```python
from build123d import *

# Parameters (mm, degrees)
SKETCH3_W           = 140
SKETCH3_H           = 140
BOSS_EXTRUDE1_DEPTH = 5
CUT_EXTRUDE1_DEPTH  = 5
CIRPATTERN1_COUNT   = 4
CUT_EXTRUDE2_REACH  = 101.121
SKETCH7_R           = 11
CIRPATTERN2_COUNT   = 4
CIRPATTERN3_COUNT   = 4


with BuildPart() as part:
    # Sketch3 → Boss-Extrude1 (new body)
    with BuildSketch(Plane.XY):
        Rectangle(SKETCH3_W, SKETCH3_H)
    extrude(amount=BOSS_EXTRUDE1_DEPTH)

    # Sketch4 → Cut-Extrude1 (cut)
    with BuildSketch(Plane.XY.offset(5)):
        with BuildLine():
            Line((7.583144073, 14.654211885), (52.928932188, 60))
            Line((52.928932188, 60), (-54.688394727, 60))
            Line((-54.688394727, 60), (-7.80758307, 14.53587447))
            ThreePointArc((-7.80758307, 14.53587447), (-0.126862728, 16.499512291), (7.583144073, 14.654211885))
        make_face()
    cut_extrude1 = extrude(amount=-CUT_EXTRUDE1_DEPTH, mode=Mode.SUBTRACT)

    # CirPattern1: Cut-Extrude1 ×4 about axis
    cirpattern1_axis = Axis((0, 0, 0), (0, 0, 1))
    for i in range(1, CIRPATTERN1_COUNT):
        add(cut_extrude1.rotate(cirpattern1_axis, i * 360 / CIRPATTERN1_COUNT), mode=Mode.SUBTRACT)

    # Sketch7 → Cut-Extrude2 (cut, up to next)
    with BuildSketch(Plane.XY.offset(5), mode=Mode.PRIVATE) as cut_extrude2_sk1:
        Circle(SKETCH7_R)
    cut_extrude2_tool1 = extrude(cut_extrude2_sk1.sketch, amount=-CUT_EXTRUDE2_REACH, mode=Mode.PRIVATE) & part.part
    add(cut_extrude2_tool1.solids().sort_by_distance((0, 0, 5))[0], mode=Mode.SUBTRACT)

    # Sketch9 → 1.8 _1.8_ Diameter Hole1 (revolve, cut)
    with BuildSketch(Plane(origin=(11.313708499, -11.313708499, 5), x_dir=(0, -1, 0), z_dir=(1, 0, 0))):
        Polygon((0, 0), (0, 6.540774557), (0.9, 6), (0.9, 0), align=None)
    f_1_8_1_8_diameter_hole1 = revolve(axis=Axis((11.313708499, -11.313708499, 11.35), (0, 0, -1)), mode=Mode.SUBTRACT)

    # CirPattern2: 1.8 _1.8_ Diameter Hole1 ×4 about axis
    cirpattern2_axis = Axis((0, 0, 0), (0, 0, 1))
    for i in range(1, CIRPATTERN2_COUNT):
        add(f_1_8_1_8_diameter_hole1.rotate(cirpattern2_axis, i * 360 / CIRPATTERN2_COUNT), mode=Mode.SUBTRACT)

    # Sketch10 → 3.0mm Dowel Hole1 (revolve, cut)
    with BuildSketch(Plane(origin=(67.5, -63, 0), x_dir=(0, 1, 0), z_dir=(1, 0, 0))):
        Polygon((0, 0), (0, 10.841204867), (1.4, 10), (1.4, 0), align=None)
    f_3_0mm_dowel_hole1 = revolve(axis=Axis((67.5, -63, -6.35), (0, 0, 1)), mode=Mode.SUBTRACT)

    # Sketch11 → 3.0mm Dowel Hole2 (revolve, cut)
    with BuildSketch(Plane(origin=(63, -67.5, 5), x_dir=(0, -1, 0), z_dir=(1, 0, 0))):
        Polygon((0, 0), (0, 10.841204867), (1.4, 10), (1.4, 0), align=None)
    f_3_0mm_dowel_hole2 = revolve(axis=Axis((63, -67.5, 11.35), (0, 0, -1)), mode=Mode.SUBTRACT)

    # CirPattern3: 3.0mm Dowel Hole1, 3.0mm Dowel Hole2 ×4 about axis
    cirpattern3_axis = Axis((0, 0, 0), (0, 0, 1))
    add([f_3_0mm_dowel_hole1.rotate(cirpattern3_axis, i * 360 / CIRPATTERN3_COUNT) for i in range(1, CIRPATTERN3_COUNT)], mode=Mode.SUBTRACT)
    add([f_3_0mm_dowel_hole2.rotate(cirpattern3_axis, i * 360 / CIRPATTERN3_COUNT) for i in range(1, CIRPATTERN3_COUNT)], mode=Mode.SUBTRACT)


solid = part.part
```
Here's how the part is built. I have some questions about the finished solid (model axes, mm). A direction names the side the tool comes from. Coordinates: 2 decimals unless noted, no trailing zeros. Order: outer loops, then holes, each group sorted by start corner. A loop starts at its lowest first (then second) coordinate and runs counter-clockwise, first axis right, second up.
Item 1: If we section it at C-C, the plane z = 3.8: Give the number of separate pieces and of enclosed holes in the cut face, then the cut area to 3 significant figures.
Response values:
separate pieces: 1
enclosed holes: 17
area: 8,070 mm2
Item 2: Which directions (+Z, -Z, +X, -X, +Y, -Y) give clear straight access to the entire face, cutting with the end or side of a thin tool? Please do faces 1 (the face through (-38, -32, 3)), 2 (the face through (70, -1, 2)).
Response values:
face 1: +Z, -Z
face 2: +Z, -Z, +X, +Y, -Y
Item 3: Thinking about a two-plate mould opening in X: for faces 3 (the face through (0, 60, 3)), 4 (the face through (-70, -1, 2)), 5 (the face through (-1, -15, 0)), which applies, pulls with the +X half, pulls with the -X half, needs draft (parallel to the pull), parting line crosses it, or undercut?
Response values:
face 3: undercut
face 4: pulls with the -X half
face 5: needs draft
Item 4: I need wall thicknesses on probe 1 along X at (y, z) = (67.5, 1.8); probe 2 along Y at (x, z) = (0, 1.9); probe 3 along X at (y, z) = (63, 1.55). Which ranges of each line are inside material? Lowest first, please.
Response values:
probe 1: x = -70 to -64.4, -61.6 to 61.6, 64.4 to 70
probe 2: y = -70 to -60, -16.5 to -11, 11 to 16.5, 60 to 70
probe 3: x = -70 to -68.9, -66.1 to 66.1, 68.9 to 70
Item 5: If we section it at A-A, the plane y = 0: List the corners of the cut face in (x, z) for me, then the cut area to 3 significant figures.
Response values:
outline: (-70, 0) - (-60, 0) - (-60, 5) - (-70, 5) - close; (-16.5, 0) - (-11, 0) - (-11, 5) - (-16.5, 5) - close; (11, 0) - (16.5, 0) - (16.5, 5) - (11, 5) - close; (60, 0) - (70, 0) - (70, 5) - (60, 5) - close
area: 155 mm2
